from build123d import *

# Parameters (mm, degrees)
PROFILEBOSS_EXTRUDE1_DEPTH                  = 33
SKETCH2_OUTSIDE_W                           = 44.01
SKETCH2_OUTSIDE_H                           = 25.28
SKETCH2_OUTSIDE_R                           = 2.5
SIDEPROFILECUT_EXTRUDE1_DEPTH               = 46.052806794
BOTTOMCUT_EXTRUDE2_DEPTH                    = 45.194291487
DRAGLINKMOUNTHOLESSKETCH4_R                 = 2
DRAGLINKMOUNTHOLESCUT_EXTRUDE3_DEPTH        = 45.194291487
CHAMFER1_SIZE                               = 1.5
CHAMFER1_SIZE2                              = 0.97411139
SKETCH4_W                                   = 4.5
SKETCH4_H                                   = 17.25
DISABLESWIIVELRESTRICTIONCUT_EXTRUDE4_DEPTH = 45.194291487


with BuildPart() as part:
    # Sketch1 → ProfileBoss-Extrude1 (new body)
    with BuildSketch(Plane(origin=(0, 0, 0), x_dir=(0, 0, -1), z_dir=(1, 0, 0))):
        Polygon((0, 14.27), (0, 0), (27.15, 0), (27.15, 14.27), (25.35, 14.27), (25.35, 3), (1.8, 3), (1.8, 14.27), align=None)
    extrude(amount=PROFILEBOSS_EXTRUDE1_DEPTH)

    # Sketch2 outside → SideProfileCut-Extrude1 (cut, through all)
    # profile 1 of 2: a face of its own
    with BuildSketch(Plane.XY):
        with Locations((16.5, 7.135)):
            Rectangle(SKETCH2_OUTSIDE_W, SKETCH2_OUTSIDE_H)
        with BuildLine():
            Line((13.093405827, 11.06), (16.093405827, 11.06))
            Line((16.093405827, 11.06), (33, 6))
            Line((33, 6), (33, 0))
            Line((33, 0), (7.135, 0))
            ThreePointArc((7.135, 0), (0.853555103, 10.519032358), (13.093405827, 11.06))
        make_face(mode=Mode.SUBTRACT)
    # profile 2 of 2: a face of its own
    with BuildSketch(Plane.XY):
        with Locations((7.135, 7.135)):
            Circle(SKETCH2_OUTSIDE_R)
    extrude(amount=-SIDEPROFILECUT_EXTRUDE1_DEPTH, mode=Mode.SUBTRACT)

    # Sketch3 → BottomCut-Extrude2 (cut, through all)
    with BuildSketch(Plane(origin=(0, 3, 0), x_dir=(1, 0, 0), z_dir=(0, 1, 0))):
        Polygon((1.320363296, 25.35), (14.55, 25.35), (14.55, 22.2), (10.05, 22.2), (10.05, 4.95), (14.55, 4.95), (14.55, 1.8), (1.320363296, 1.8), align=None)
    extrude(amount=-BOTTOMCUT_EXTRUDE2_DEPTH, mode=Mode.SUBTRACT)

    # DragLinkMountHolesSketch4 → DragLinkMountHolesCut-Extrude3 (cut, through all)
    with BuildSketch(Plane(origin=(0, 3, 0), x_dir=(1, 0, 0), z_dir=(0, 1, 0))):
        with Locations(Location((28, 19.575, 0), (0, 0, 270))):
            Circle(DRAGLINKMOUNTHOLESSKETCH4_R)
        with Locations(Location((28, 7.575, 0), (0, 0, 270))):
            Circle(DRAGLINKMOUNTHOLESSKETCH4_R)
        with Locations(Location((20.5, 13.575, 0), (0, 0, 270))):
            Circle(DRAGLINKMOUNTHOLESSKETCH4_R)
    extrude(amount=-DRAGLINKMOUNTHOLESCUT_EXTRUDE3_DEPTH, mode=Mode.SUBTRACT)

    # Chamfer1
    chamfer1_edges = [part.edges().sort_by_distance(p)[0] for p in [
        (28, 3, -21.575),
        (28, 3, -9.575),
        (20.5, 3, -15.575),
    ]]
    chamfer1_side = [part.faces().sort_by_distance(p)[0] for p in [
        (14.878832024, 3, -23.775),
    ]]
    chamfer(chamfer1_edges, length=CHAMFER1_SIZE, length2=CHAMFER1_SIZE2, reference=chamfer1_side[0])

    # Sketch4 → DisableSwiivelRestrictionCut-Extrude4 (cut, through all)
    with BuildSketch(Plane(origin=(0, 3, 0), x_dir=(1, 0, 0), z_dir=(0, 1, 0))):
        with Locations((12.3, 13.575)):
            Rectangle(SKETCH4_W, SKETCH4_H)
    extrude(amount=-DISABLESWIIVELRESTRICTIONCUT_EXTRUDE4_DEPTH, mode=Mode.SUBTRACT)


solid = part.part
Work out the finished part from the listing and answer in its coordinate system (mm). A direction names the side the tool comes from. Give positions to 0.01 mm unless a question says otherwise; leave off trailing zeros. Loops run counter-clockwise (first coordinate to the right, second up) from the corner with the lowest first, then second, coordinate; pieces in that order, holes last. Notation, with made-up numbers: (-17, -10) - (25, -10) arc R3 cw to (25, -6) - close; hole circle Ø1 at (46.25, 77.25). An arc over 180 degrees is marked (long way). Answer in a Markdown table with one row per item.
(1) Section C-C (x = 20.5) is taken. Give the vertices of the cut face in (y, z) (3 decimals), and give its area (3 significant figures).
Results list:
| item | result |
|---|---|
| outline | (0, -27.15) - (9.741, -27.15) - (9.741, -25.35) - (3, -25.35) - (3, -17.075) - (2.026, -15.575) - (0, -15.575) - close; (0, -11.575) - (2.026, -11.575) - (3, -10.075) - (3, -1.8) - (9.741, -1.8) - (9.741, 0) - (0, 0) - close |
| area | 92.3 mm² |
(2) Section D-D (y = 3.5) is taken. Give the vertices of the cut face in (x, z), and give its area (3 significant figures).
Results list:
| item | result |
|---|---|
| outline | (1, -27.15) - (33, -27.15) - (33, -25.35) - (1, -25.35) - close; (1, -1.8) - (33, -1.8) - (33, 0) - (1, 0) - close |
| area | 115 mm² |
(3) Flat-ended cylindrical pins translate along their axes: pin 1 Ø1.5 at (y, z) = (3.5, -20) entering from -X; pin 2 Ø2 at (x, z) = (15.5, -26) entering from +Y; pin 3 Ø12 at (x, z) = (9.5, -8.5) entering from +Y. Find the tip coordinate at first contact, or state that the pin passes through.
Results list:
| item | result |
|---|---|
| pin 1 | stops at x = 14.55 |
| pin 2 | stops at y = 11.06 |
| pin 3 | stops at y = 3 |
(4) Consider L1, parallel to Z at x = 28.5, y = 4.75; L2, parallel to Y at x = 19, z = -18; L3, parallel to X at y = 2.25, z = -13.5. Determine where each line is inside the solid, lowest interval first. Write a range as [from, to].
Results list:
| item | result |
|---|---|
| L1 | z = [-27.15, -25.35], [-1.8, 0] |
| L2 | y = [0, 3] |
| L3 | x = [14.55, 18.16], [22.84, 33] |
(5) A tool of negligible diameter and unlimited length cuts with its end or side. For faces 5 (the face through (6.593, 4.694, -26.237)), 6 (the face through (15, 11.06, -1)), 7 (the face through (16, 5, -27.15)), 8 (the face through (13, 7, -1.8)), 9 (the face through (26, 3, -14)), from which of +Z, -Z, +X, -X, +Y, -Y can it reach the whole face along a straight path? Write none if from no direction.
Results list:
| item | result |
|---|---|
| face 5 | +Z, -Z |
| face 6 | +Z, -Z, +X, +Y |
| face 7 | -Z, +X, -X, +Y, -Y |
| face 8 | -X, +Y |
| face 9 | +X, -X, +Y |
(6) Section A-A (y = 12) is taken. Give the vertices of the cut face in (x, z), and give its area (3 significant figures).
Results list:
| item | result |
|---|---|
| outline | (1.92, -27.15) - (12.35, -27.15) - (12.35, -25.35) - (1.92, -25.35) - close; (1.92, -1.8) - (12.35, -1.8) - (12.35, 0) - (1.92, 0) - close |
| area | 37.6 mm² |
(7) For a pull along X with two mould halves and no side action, classify faces 1 (the face through (13, 7, -25.35)), 2 (the face through (26.78, 1.03, -21.16)), 3 (the face through (0.76, 10.34, -0.89)), 4 (the face through (24.428, 8.565, -0.887)) as pulls with the +X half, pulls with the -X half, needs draft (parallel to the pull), parting line crosses it, or undercut.
Results list:
| item | result |
|---|---|
| face 1 | needs draft |
| face 2 | undercut |
| face 3 | parting line crosses it |
| face 4 | pulls with the +X half |
(8) Section B-B (x = 28) is taken. Give the vertices of the cut face in (y, z) (3 decimals), and give its area (3 significant figures).
Results list:
| item | result |
|---|---|
| outline | (0, -27.15) - (7.496, -27.15) - (7.496, -25.35) - (3, -25.35) - (3, -23.075) - (2.026, -21.575) - (0, -21.575) - close; (0, -17.575) - (2.026, -17.575) - (3, -16.075) - (3, -11.075) - (2.026, -9.575) - (0, -9.575) - close; (0, -5.575) - (2.026, -5.575) - (3, -4.075) - (3, -1.8) - (7.496, -1.8) - (7.496, 0) - (0, 0) - close |
| area | 70.7 mm² |
